Design review of the part built by this model. Coordinates are the model's own, in mm. A direction names the side the tool comes from. Round coordinates to 2 decimals unless told otherwise and drop trailing zeros. Loops run counter-clockwise (first coordinate to the right, second up) from the corner with the lowest first, then second, coordinate; pieces in that order, holes last. Notation, with made-up numbers: (-13.75, -13) -> (10.25, -13) arc R30 cw to (10.25, 12) -> close; hole circle Ø4 at (-8.5, 48.25). An arc over 180 degrees is marked (long way). Use a Markdown table: item, result. Add a question column.
Autodesk Inventor part; units mm, degrees
ref_plane "YZ Plane" through (0, 0, 0) normal (1, 0, 0) x (0, 1, 0)
ref_plane "XZ Plane" through (0, 0, 0) normal (0, 1, 0) x (-1, 0, 0)
ref_plane "XY Plane" through (0, 0, 0) normal (0, 0, 1) x (1, 0, 0)
sketch "Эскиз1" plane through (0, 0, 0) normal (0, 0, 1) x (1, 0, 0)
  line L0 (0, 0) -> (60, 0)
  line L1 (60, 0) -> (60, -100)
  line L2 (60, -100) -> (0, -100)
  line L3 (0, -100) -> (0, 0)
  line L4 (2, -2) -> (58, -2)
  line L5 (58, -2) -> (58, -98)
  line L6 (58, -98) -> (2, -98)
  line L7 (2, -98) -> (2, -2)
  line L8 (0, 0) -> (60, -100) construction
  line L9 (60, 0) -> (0, -100) construction
  line L10 (2, -2) -> (58, -98) construction
  line L11 (58, -2) -> (2, -98) construction
  line L12 (20, -15) -> (40, -15)
  line L13 (40, -15) -> (40, -85)
  line L14 (40, -85) -> (20, -85)
  line L15 (20, -85) -> (20, -15)
  line L16 (20, -15) -> (40, -85) construction
  line L17 (40, -15) -> (20, -85) construction
  point P0 (30, -50)
  point P1 (30, -50)
  dimension "d0" = 60
  dimension "d1" = 100
  dimension "d2" = 56
  dimension "d3" = 96
  dimension "d8" = 20
  dimension "d9" = 70
extrude "Выдавливание1" add sketch "Эскиз1" along normal blind 30 contours L0 L1 L2 L3 | L4 L5 L6 L7 | L12 L13 L14 L15
extrude "Выдавливание2" cut sketch "Эскиз1" along normal blind 28 contours L4 L5 L6 L7 | L12 L13 L14 L15
extrude "Выдавливание3" add sketch "Эскиз1" along normal blind 30 contours L12 L13 L14 L15
extrude "Выдавливание4" cut sketch "Эскиз1" along normal blind 35 contours L12 L13 L14 L15
sketch "Эскиз2" plane through (0, 0, 0) normal (0, 1, 0) x (-1, 0, 0)
  line L0 (-60, 0) -> (-60, 30)
  line L1 (-60, 30) -> (0, 30)
  line L2 (-60, 0) -> (0, 30) construction
  line L3 (-60, 0) -> (0, 0)
  line L4 (-60, 30) -> (0, 0) construction
  line L5 (-37.5, 20) -> (-22.5, 20)
  line L6 (-22.5, 20) -> (-22.5, 10)
  line L7 (-22.5, 10) -> (-37.5, 10)
  line L8 (-37.5, 10) -> (-37.5, 20)
  line L9 (-37.5, 20) -> (-22.5, 10) construction
  line L10 (-22.5, 20) -> (-37.5, 10) construction
  circle A0 centre (-30, 15) radius 2.5
  dimension "d14" = 15
  dimension "d15" = 10
  dimension "d16" = 5
extrude "Выдавливание5" cut sketch "Эскиз2" along normal mid plane 100 contours L5 L6 L7 L8 | A0
extrude "Выдавливание6" cut sketch "Эскиз2" against normal through all contours A0
extrude "Выдавливание9" add sketch "Эскиз1" along normal blind 2 contours L0 L1 L2 L3 | L4 L5 L6 L7 | L12 L13 L14 L15
properties part number "Корпус" material "Полиацеталь, черный"
1. For faces 5 (the face through (32.5, -99, 15.1)), 6 (the face through (40, -50, 29)), 7 (the face through (30, -2, 9)), 8 (the face through (30, -1, 20)), 9 (the face through (30, -100, 11)), list the 3-axis set-ups (+Z, -Z, +X, -X, +Y, -Y) from which the entire face can be reached by the end or side of a thin tool; tool diameter is ignored.
2. To check wall thickness, follow probe 1 along Z at (x, y) = (50.5, -38); probe 2 along Z at (x, y) = (30, -99); probe 3 along Y at (x, z) = (15.5, 23.5). State the ranges of each line that lie inside material, in increasing order. Write a range as from..to.
3. Consider section A-A on x = 30. State the section outline as (y, z) points.
4. Consider section D-D on z = 3. State the section outline as (x, y) points, plus the area to 3 significant figures.
5. Consider section C-C on y = -46.5. State the section outline as (x, z) points.
6. Mouldability with a two-part tool opening along X and no side actions: class faces 1 (the face through (0, -51, 15)), 2 (the face through (30, -15, 29)), 3 (the face through (37.5, -1, 15)), 4 (the face through (16, -49, 30)) as +X half, -X half, draft (parallel to the pull), parting line (faces both ways), or undercut.
7. Consider section B-B on z = 11.5. State the section outline as (x, y) points.
Verdict:
| question | item | result |
|---|---|---|
| 1 | face 5 | +Y, -Y |
| 1 | face 6 | +Z |
| 1 | face 7 | none |
| 1 | face 8 | +Y |
| 1 | face 9 | +Z, -Z, +X, -X, -Y |
| 2 | probe 1 | z = 0..2, 28..30 |
| 2 | probe 2 | z = 0..12.5, 17.5..30 |
| 2 | probe 3 | y = -100..-98, -2..0 |
| 3 | outline | (-100, 0) -> (0, 0) -> (0, 10) -> (-2, 10) -> (-2, 2) -> (-98, 2) -> (-98, 12.5) -> (-100, 12.5) -> close; (-100, 17.5) -> (-98, 17.5) -> (-98, 28) -> (-85, 28) -> (-85, 30) -> (-100, 30) -> close; (-15, 28) -> (-2, 28) -> (-2, 20) -> (0, 20) -> (0, 30) -> (-15, 30) -> close |
| 4 | outline | (0, -100) -> (60, -100) -> (60, 0) -> (0, 0) -> close; hole (2, -98) -> (58, -98) -> (58, -2) -> (2, -2) -> close |
| 4 | area | 624 mm² |
| 5 | outline | (0, 0) -> (60, 0) -> (60, 30) -> (40, 30) -> (40, 28) -> (58, 28) -> (58, 2) -> (2, 2) -> (2, 28) -> (20, 28) -> (20, 30) -> (0, 30) -> close |
| 6 | face 1 | -X half |
| 6 | face 2 | undercut |
| 6 | face 3 | undercut |
| 6 | face 4 | draft |
| 7 | outline | (0, -100) -> (60, -100) -> (60, 0) -> (37.5, 0) -> (37.5, -2) -> (58, -2) -> (58, -98) -> (2, -98) -> (2, -2) -> (22.5, -2) -> (22.5, 0) -> (0, 0) -> close |
